Geometry check sheet. Reference: the model listing, model coordinates, mm. A direction names the side the tool comes from. Round coordinates to 2 decimals unless told otherwise and drop trailing zeros. Order: outer loops, then holes, each group sorted by start corner. A loop starts at its lowest first (then second) coordinate and runs counter-clockwise, first axis right, second up.
(1) Sectioned sample at A-A (z = -25.4). Record the boundary of the cut face in (x, y), plus the area to 3 significant figures.
(2) Sectioned sample at B-B (x = -116). Record the boundary of the cut face in (y, z).
(3) Release check for a two-part mould opening along Z. For faces 4 (the face through (193.957, -5, 1)), 5 (the face through (170.288, -5.134, 27.803)), 6 (the face through (2, -72, -91.44)), 7 (the face through (170.288, -5.134, -22.997)) record: +Z half, -Z half, draft (parallel to the pull), parting line (faces both ways), or undercut.
(4) Material ranges on line 1 along X through (y, z) = (-3.75, -25.4); line 2 along Z through (x, y) = (61.5, -126.5); line 3 along X through (y, z) = (-133, -14.5), recorded low to high.
(5) Set-up check for faces 1 (the face through (-170.288, -5.134, -73.797)), 2 (the face through (3.212, -146.015, 6.431)), 3 (the face through (173, -10.414, 1)): record each of +Z, -Z, +X, -X, +Y, -Y from which the full face is reachable in a straight line by a thin tool's end or side.
(6) Sectioned sample at C-C (y = -49). Record the boundary of the cut face in (x, z), plus the area to 3 significant figures.
(7) Go/stop test with flat-tipped pins: pin 1 (3 mm diameter, centred on y = -143, z = 38, fed in from +X); pin 2 (1 mm diameter, centred on x = -132.5, z = -75.5, fed in from +Y); pin 3 (1 mm diameter, centred on x = -102, z = 27, fed in from +Y). Record where each tip stops, or that it passes through.
(8) Sectioned sample at D-D (z = -62.5). Record the boundary of the cut face in (x, y), plus the area to 3 significant figures.
from build123d import *

# Parameters (mm, degrees)
BOSS_EXTRUDE1_DEPTH = 101.6
CUT_EXTRUDE1_DEPTH  = 193.04
CUT_EXTRUDE2_DEPTH  = 320.596404315
SKETCH5_R           = 5.207
CUT_EXTRUDE4_DEPTH  = 82.042


with BuildPart() as part:
    # Sketch2 → Boss-Extrude1 (new, symmetric)
    with BuildSketch(Plane.XY):
        with BuildLine():
            Line((-187.042762313, 0), (193.957237687, 0))
            Line((193.957237687, 0), (193.957237687, -10.414))
            Line((193.957237687, -10.414), (152.043772, -10.414))
            ThreePointArc((152.043772, -10.414), (131.741592603, -76.615356022), (84.242269675, -127))
            Line((84.242269675, -127), (177.8, -127))
            Line((177.8, -127), (177.8, -165.1))
            Line((177.8, -165.1), (-177.8, -165.1))
            Line((-177.8, -165.1), (-177.8, -127))
            Line((-177.8, -127), (-84.242269675, -127))
            ThreePointArc((-84.242269675, -127), (-131.741592603, -76.615356022), (-152.043772, -10.414))
            Line((-152.043772, -10.414), (-187.042762313, -10.414))
            Line((-187.042762313, -10.414), (-187.042762313, 0))
        make_face()
    extrude(amount=BOSS_EXTRUDE1_DEPTH, both=True)

    # Sketch3 → Cut-Extrude1 (cut)
    with BuildSketch(Plane.XY.offset(101.6)):
        with BuildLine():
            Line((-146.05, 0), (146.05, 0))
            ThreePointArc((146.05, 0), (0, -146.05), (-146.05, 0))
        make_face()
    extrude(amount=-CUT_EXTRUDE1_DEPTH, mode=Mode.SUBTRACT)

    # Sketch4 → Cut-Extrude2 (cut, through all)
    with BuildSketch(Plane.XY.offset(-91.44)):
        with BuildLine():
            Line((-38.1, 0), (38.1, 0))
            ThreePointArc((38.1, 0), (0, -38.1), (-38.1, 0))
        make_face()
    extrude(amount=-CUT_EXTRUDE2_DEPTH, mode=Mode.SUBTRACT)

    # Sketch5 → Cut-Extrude4 (cut)
    with BuildSketch(Plane(origin=(0, 0, 0), x_dir=(1, 0, 0), z_dir=(0, 1, 0))):
        with Locations(Location((174.907237687, -76.2, 0), (0, 0, 270))):
            Circle(SKETCH5_R)
        with Locations(Location((174.907237687, -25.4, 0), (0, 0, 270))):
            Circle(SKETCH5_R)
        with Locations(Location((174.907237687, 25.4, 0), (0, 0, 270))):
            Circle(SKETCH5_R)
        with Locations(Location((174.907237687, 76.2, 0), (0, 0, 270))):
            Circle(SKETCH5_R)
    cut_extrude4 = extrude(amount=-CUT_EXTRUDE4_DEPTH, mode=Mode.SUBTRACT)

    # Mirror1: Cut-Extrude4 across plane
    add(cut_extrude4.mirror(Plane(origin=(0, 0, 0), x_dir=(0, 0, 1), z_dir=(1, 0, 0))), mode=Mode.SUBTRACT)


solid = part.part
Answer below:
1. outline: (-187.04, -10.41) - (-180.11, -10.41) - (-180.11, 0) - (-187.04, 0) - close; (-177.8, -165.1) - (177.8, -165.1) - (177.8, -127) - (84.24, -127) arc R152.4 ccw to (152.04, -10.41) - (169.7, -10.41) - (169.7, 0) - (146.05, 0) arc R146.05 cw to (-146.05, 0) - (-169.7, 0) - (-169.7, -10.41) - (-152.04, -10.41) arc R152.4 ccw to (-84.24, -127) - (-177.8, -127) - close; (180.11, -10.41) - (193.96, -10.41) - (193.96, 0) - (180.11, 0) - close
1. area: 14,200 mm2
2. outline: (-165.1, -101.6) - (-127, -101.6) - (-127, 101.6) - (-165.1, 101.6) - close; (-98.84, -101.6) - (0, -101.6) - (0, -91.44) - (-88.74, -91.44) - (-88.74, 101.6) - (-98.84, 101.6) - close
3. face 4: draft
3. face 5: undercut
3. face 6: +Z half
3. face 7: undercut
4. line 1: x = -187.04 to -180.11, -169.7 to -146, 146 to 169.7, 180.11 to 193.96
4. line 2: z = -101.6 to -91.44
4. line 3: x = -177.8 to -60.35, 60.35 to 177.8
5. face 1: +Y
5. face 2: +Z, +Y
5. face 3: +Z, -Z, +X
6. outline: (-144.31, -101.6) - (144.31, -101.6) - (144.31, 101.6) - (137.58, 101.6) - (137.58, -91.44) - (-137.58, -91.44) - (-137.58, 101.6) - (-144.31, 101.6) - close
6. area: 5,530 mm2
7. pin 1: stops at x = 177.8
7. pin 2: stops at y = -60.35
7. pin 3: stops at y = -104.04
8. outline: (-187.04, -10.41) - (-152.04, -10.41) arc R152.4 ccw to (-84.24, -127) - (-177.8, -127) - (-177.8, -165.1) - (177.8, -165.1) - (177.8, -127) - (84.24, -127) arc R152.4 ccw to (152.04, -10.41) - (193.96, -10.41) - (193.96, 0) - (146.05, 0) arc R146.05 cw to (-146.05, 0) - (-187.04, 0) - close
8. area: 14,400 mm2
